Part model, mm, in its own coordinate system. Face numbers are marked on the shaded views. A direction names the side the tool comes from. Give positions to 0.01 mm unless a question says otherwise; leave off trailing zeros. Write each loop counter-clockwise with the first axis right and the second up, starting at its lowest first coordinate (ties: lowest second). Pieces come first, ordered by that corner, then holes.
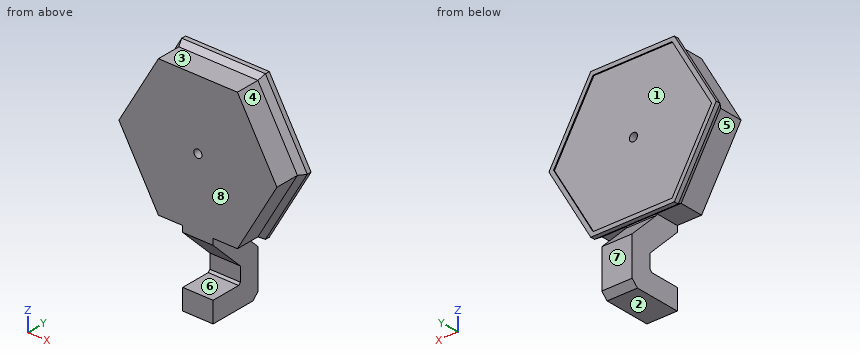
```python
from build123d import *

# Parameters (mm, degrees)
SALIENTE_EXTRUIR1_DEPTH = 11.8
SALIENTE_EXTRUIR2_DEPTH = 2.2
CORTAR_EXTRUIR1_DEPTH   = 0.5
CROQUIS7_R              = 2
CORTAR_EXTRUIR2_DEPTH   = 58.071950338
SALIENTE_EXTRUIR3_DEPTH = 7.5


with BuildPart() as part:
    # Croquis1 → Saliente-Extruir1 (new body)
    with BuildSketch(Plane(origin=(0, 0, 0), x_dir=(1, 0, 0), z_dir=(0, 1, 0))):
        Polygon((19.5, -33.774990748), (39, 0), (19.5, 33.774990748), (-19.5, 33.774990748), (-39, 0), (-19.5, -33.774990748), align=None)
    extrude(amount=SALIENTE_EXTRUIR1_DEPTH)

    # Croquis4 → section 1 of recubrir2
    with BuildSketch(Plane(origin=(0, 14.8, 0), x_dir=(1, 0, 0), z_dir=(0, 1, 0)), mode=Mode.PRIVATE) as recubrir2_s1:
        with BuildLine():
            Line((20.65, -35.766849176), (41.3, 0))
            Line((41.3, 0), (20.65, 35.766849176))
            Line((20.65, 35.766849176), (-20.65, 35.766849176))
            Line((-20.65, 35.766849176), (-41.3, 0))
            Line((-41.3, 0), (-20.65, -35.766849176))
            Line((-20.65, -35.766849176), (20.65, -35.766849176))
        make_face()
    # loft from a face of the part (recubrir2)
    loft([part.faces().sort_by_distance((0, 11.8, 0))[0], recubrir2_s1.sketch])

    # Croquis5 → Saliente-Extruir2 (add)
    with BuildSketch(Plane(origin=(0, 14.8, 0), x_dir=(1, 0, 0), z_dir=(0, 1, 0))):
        Polygon((20.65, -35.766849176), (41.3, 0), (20.65, 35.766849176), (-20.65, 35.766849176), (-41.3, 0), (-20.65, -35.766849176), align=None)
    extrude(amount=SALIENTE_EXTRUIR2_DEPTH)

    # Croquis6 → Cortar-Extruir1 (cut)
    with BuildSketch(Plane(origin=(0, 17, 0), x_dir=(1, 0, 0), z_dir=(0, 1, 0))):
        Polygon((19.5, -33.774990748), (39, 0), (19.5, 33.774990748), (-19.5, 33.774990748), (-39, 0), (-19.5, -33.774990748), align=None)
    extrude(amount=-CORTAR_EXTRUIR1_DEPTH, mode=Mode.SUBTRACT)

    # Croquis7 → Cortar-Extruir2 (cut, through all)
    with BuildSketch(Plane(origin=(0, 16.5, 0), x_dir=(1, 0, 0), z_dir=(0, 1, 0))):
        with Locations(Location((0, 0, 0), (0, 0, 270))):
            Circle(CROQUIS7_R)
    extrude(amount=-CORTAR_EXTRUIR2_DEPTH, mode=Mode.SUBTRACT)

    # Croquis8 → Saliente-Extruir3 (add, symmetric)
    with BuildSketch(Plane(origin=(0, 0, 0), x_dir=(0, 0, -1), z_dir=(1, 0, 0))):
        Polygon((36.774990748, 0), (52.47276129, 15.697770542), (59.47276129, 15.697770542), (60.469781851, 14.700749981), (60.469781851, 0), (70.716946405, 0), (70.716946405, 22.948703413), (67.771594914, 25.998704166), (48.631594914, 25.998704166), (34.432890748, 11.8), (33.774990748, 11.8), (33.774990748, 0), align=None)
    extrude(amount=SALIENTE_EXTRUIR3_DEPTH, both=True)


solid = part.part
```
1) Saw through at A-A, the plane y = 7. Write the cut outline in (x, z) (3 decimals).
Answers follow:
outline: (-39, 0) - (-19.5, -33.775) - (-7.5, -33.775) - (-7.5, -43.775) - (7.5, -43.775) - (7.5, -33.775) - (19.5, -33.775) - (39, 0) - (19.5, 33.775) - (-19.5, 33.775) - close; (-7.5, -70.717) - (7.5, -70.717) - (7.5, -60.47) - (-7.5, -60.47) - close; hole circle Ø4 at (0, 0)
2) Pin check, flat tips, straight feed: pin 1 Ø2 at (x, y) = (6.5, 8) entering from +Z (3 decimals); pin 2 Ø12 at (x, y) = (3, 8) entering from +Z; pin 3 Ø13 at (x, y) = (-14.5, 3) entering from -Z (3 decimals). Stop position of each tip, or through.
Answers follow:
pin 1: stops at z = 33.775
pin 2: stops at z = 35.24
pin 3: stops at z = -33.775
3) Wall check: L1, parallel to Z at x = 4.5, y = 15.25 (3 decimals); L2, parallel to X at y = 9.25, z = 0; L3, parallel to Y at x = -21, z = 8. Give the ranges that are in metal, low to high.
Answers follow:
L1: z = -70.717 to -59.921, -52.025 to -37.883, -35.767 to 35.767
L2: x = -39 to -2, 2 to 39
L3: y = 0 to 16.5
4) Saw through at B-B, the plane z = -54. Write the cut outline in (x, y).
Answers follow:
outline: (-7.5, 15.7) - (7.5, 15.7) - (7.5, 26) - (-7.5, 26) - close
5) 3-axis set-ups, long thin cutter, end or side, ignore diameter. For the marked faces 4, 5, 6, 7 and 8: which of +Z, -Z, +X, -X, +Y, -Y reach the whole face in a straight line?
Answers follow:
face 4: +Z, +X, -Y
face 5: -Z, -X, -Y
face 6: +X, -X, -Y
face 7: +Z, -Z, +X, -X, +Y
face 8: +Z, -Z, +X, -X, -Y
6) Two-plate mould, pull along Z, no slides. Class the marked faces 1, 2 and 3: +Z half, -Z half, draft (parallel to the pull), parting line (faces both ways), or undercut.
Answers follow:
face 1: undercut
face 2: -Z half
face 3: +Z half
